The listing builds one solid part. Answer for the finished solid, in the listing's coordinates (mm). A direction names the side the tool comes from. Coordinates: 2 decimals unless noted, no trailing zeros. Loops run counter-clockwise (first coordinate to the right, second up) from the corner with the lowest first, then second, coordinate; pieces in that order, holes last. Notation, with made-up numbers: (84, -36) - (106, -36) arc R23 cw to (106, -20) - close; hole circle Ø7 at (66.25, 28.25). An arc over 180 degrees is marked (long way). Return JSON: item names as keys, results as strings. Group by question number.
1. Which of the six approach directions +Z, -Z, +X, -X, +Y, -Y give full straight-line access (tool end or side, diameter ignored) to faces 4 (the face through (201.568, 293.967, 50.089)), 5 (the face through (202.769, 296.206, 50.089))?
2. Section B-B (x = 25) is taken. Write down the section's boundary in (y, z).
3. Each of these flat-tipped pins is pushed along its axis until it touches: P1, Ø10, axis at x = 100.5, z = 52.5, coming from the -Y side; P2, Ø12, axis at y = 133, z = 85.5, coming from the -X side; P3, Ø1.5, axis at x = 45, z = 16, coming from the -Y side. Where does it stop, or does it pass through?
4. Section C-C (z = 10) is taken. Write down the section's boundary in (x, y).
5. The mould has two halves that part along Y. Classify faces 1 (the face through (96, 272, 0)), 2 (the face through (211.2, 274.7, 50.1)), 3 (the face through (221.157, 243.253, 50.089)): pulls with the +Y half, pulls with the -Y half, needs draft (parallel to the pull), parting line crosses it, or undercut.
6. Find the intervals of material crossed by line 1 along X through (y, z) = (245.5, 85); line 2 along Y through (x, z) = (166.5, 14); line 3 along Y through (x, z) = (52, 59.5), in increasing order.
7. Section A-A (y = 246.5) is taken. Write down the section's boundary in (x, z).
```python
from build123d import *

# Parameters (mm, degrees)
BOSS_EXTRUDE1_DEPTH = 101.6


with BuildPart() as part:
    # Sketch1 → Boss-Extrude1 (new body)
    with BuildSketch(Plane.XY):
        with BuildLine():
            Line((51.799660555, 261.122372087), (197.186615042, 299.043929939))
            Line((197.186615042, 299.043929939), (208.509660322, 293.287113842))
            Line((208.509660322, 293.287113842), (218.620076974, 258.056123915))
            ThreePointArc((218.620076974, 258.056123915), (221.169715366, 243.040079022), (220.342179316, 227.83161282))
            Line((220.342179316, 227.83161282), (215.6257762, 199.617635489))
            ThreePointArc((215.6257762, 199.617635489), (198.699129745, 155.371015972), (165.895883475, 121.19175716))
            Line((165.895883475, 121.19175716), (135.007693071, 99.777817102))
            ThreePointArc((135.007693071, 99.777817102), (73.443869598, 84.610101156), (17.431420723, 114.321538997))
            Line((17.431420723, 114.321538997), (17.036655023, 114.773038812))
            ThreePointArc((17.036655023, 114.773038812), (5.027038746, 135.249887254), (1.376775545, 158.7063956))
            Line((1.376775545, 158.7063956), (2.687868659, 197.659197646))
            ThreePointArc((2.687868659, 197.659197646), (16.992541419, 237.323825473), (51.799660555, 261.122372087))
        make_face()
        with BuildLine():
            Line((52.480544155, 258.674987582), (196.894837031, 296.342844243))
            Line((196.894837031, 296.342844243), (206.373128662, 291.523930207))
            Line((206.373128662, 291.523930207), (216.178620917, 257.355486833))
            ThreePointArc((216.178620917, 257.355486833), (218.633828258, 242.895591751), (217.836941691, 228.250402074))
            Line((217.836941691, 228.250402074), (213.120538575, 200.036424744))
            ThreePointArc((213.120538575, 200.036424744), (196.554033533, 156.731222664), (164.448728673, 123.279182124))
            Line((164.448728673, 123.279182124), (133.560538269, 101.865242067))
            ThreePointArc((133.560538269, 101.865242067), (73.755681182, 87.130889432), (19.343587989, 115.99342905))
            Line((19.343587989, 115.99342905), (18.948822289, 116.444928865))
            ThreePointArc((18.948822289, 116.444928865), (7.419590663, 136.102703369), (3.91533799, 158.620951381))
            Line((3.91533799, 158.620951381), (5.226431104, 197.573753427))
            ThreePointArc((5.226431104, 197.573753427), (18.98894665, 235.75335118), (52.480544155, 258.674987582))
        make_face(mode=Mode.SUBTRACT)
    extrude(amount=BOSS_EXTRUDE1_DEPTH)


solid = part.part
```
The answers:
{
 "1": {"face 4": "+Z, -Z", "face 5": "+Z, -Z, +X, +Y"},
 "2": {"outline": "(106.66, 0) - (110.11, 0) - (110.11, 101.6) - (106.66, 101.6) - close; (242.51, 0) - (246.01, 0) - (246.01, 101.6) - (242.51, 101.6) - close"},
 "3": {"P1": "stops at y = 84.64", "P2": "stops at x = 3.82", "P3": "stops at y = 92.76"},
 "4": {"outline": "(1.38, 158.71) arc R63.5 ccw to (17.04, 114.77) - (17.43, 114.32) arc R88.9 ccw to (135.01, 99.78) - (165.9, 121.19) arc R119.38 ccw to (215.63, 199.62) - (220.34, 227.83) arc R68.58 ccw to (218.62, 258.06) - (208.51, 293.29) - (197.19, 299.04) - (51.8, 261.12) arc R68.58 ccw to (2.69, 197.66) - close; hole (3.92, 158.62) arc R60.96 ccw to (18.95, 116.44) - (19.34, 115.99) arc R86.36 ccw to (133.56, 101.87) - (164.45, 123.28) arc R116.84 ccw to (213.12, 200.04) - (217.84, 228.25) arc R66.04 ccw to (216.18, 257.36) - (206.37, 291.52) - (196.89, 296.34) - (52.48, 258.67) arc R66.04 ccw to (5.23, 197.57) - close"},
 "5": {"face 1": "needs draft", "face 2": "undercut", "face 3": "parting line crosses it"},
 "6": {"line 1": "x = 24.45 to 28.26, 218.43 to 220.99", "line 2": "y = 121.61 to 124.73, 288.41 to 291.04", "line 3": "y = 90.04 to 92.77, 258.53 to 261.17"},
 "7": {"outline": "(25.54, 0) - (29.45, 0) - (29.45, 101.6) - (25.54, 101.6) - close; (218.33, 0) - (220.88, 0) - (220.88, 101.6) - (218.33, 101.6) - close"}
}
